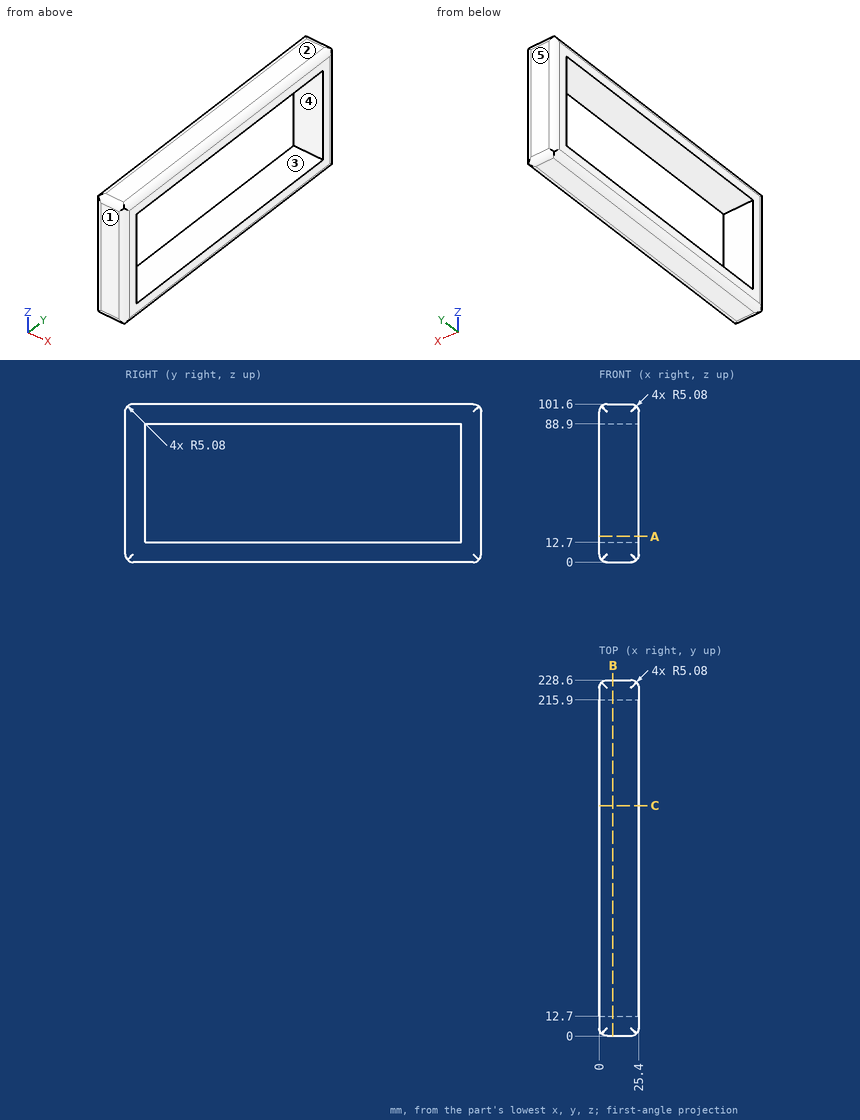
Verification items for this drawing (mm, ordinates from the low corner). A direction names the side the tool comes from. Give positions to 0.01 mm unless a question says otherwise; leave off trailing zeros. Loops run counter-clockwise (first coordinate to the right, second up) from the corner with the lowest first, then second, coordinate; pieces in that order, holes last. Notation, with made-up numbers: M 23,11.25 L 72,11.25 A7 cw 72,23.25 Z; hole C 77,58.5 d10. An arc over 180 degrees is marked long. Write item = value, one per line. Start each with the question number.
1. Tool access check on the marked faces 4 and 5. Record the directions out of +Z, -Z, +X, -X, +Y, -Y that give a thin tool (end or side, any length) a straight path to the whole face; none if there is none.
2. Section check A-A, the plane z = 16.5. Enter the section's corners in (x, y).
3. Section check C-C, the plane y = 148. Enter the section's corners in (x, z).
4. Thickness scan on probe 1 along Z at (x, y) = (15, 73); probe 2 along Y at (x, z) = (9.75, 32); probe 3 along Z at (x, y) = (23, 23). Record the ranges inside material, lowest first.
5. Draft check along Y on the marked faces 1, 2 and 3. Enter one of: +Y half, -Y half, draft (parallel to the pull), parting line (faces both ways), or undercut.
6. Go/stop test with a flat-tipped pin: P1, Ø1, axis at x = 22.5, y = 154, coming from the -Z side. Record where the tip stops, or that it passes through.
7. Section check B-B, the plane x = 8.75. Enter the section's corners in (y, z).
Values follow:
q1.face_4 = +X, -X
q1.face_5 = +Z, -Z, +X, -X, +Y
q2.outline = M 0,5.08 A5.08 ccw 5.08,0 L 20.32,0 A5.08 ccw 25.4,5.08 L 25.4,12.7 L 0,12.7 Z; M 0,215.9 L 25.4,215.9 L 25.4,223.52 A5.08 ccw 20.32,228.6 L 5.08,228.6 A5.08 ccw 0,223.52 Z
q3.outline = M 0,5.08 A5.08 ccw 5.08,0 L 20.32,0 A5.08 ccw 25.4,5.08 L 25.4,12.7 L 0,12.7 Z; M 0,88.9 L 25.4,88.9 L 25.4,96.52 A5.08 ccw 20.32,101.6 L 5.08,101.6 A5.08 ccw 0,96.52 Z
q4.probe_1 = 0 to 12.7, 88.9 to 101.6
q4.probe_2 = 0 to 12.7, 215.9 to 228.6
q4.probe_3 = 0.76 to 12.7, 88.9 to 100.84
q5.face_1 = -Y half
q5.face_2 = draft
q5.face_3 = undercut
q6.P1 = 0.29
q7.outline = M 0,5.08 A5.08 ccw 5.08,0 L 223.52,0 A5.08 ccw 228.6,5.08 L 228.6,96.52 A5.08 ccw 223.52,101.6 L 5.08,101.6 A5.08 ccw 0,96.52 Z; hole M 12.7,12.7 L 215.9,12.7 L 215.9,88.9 L 12.7,88.9 Z
